Design review of the part shown in the three views and the two pictorial views. Dimensions are in mm from the part's minimum x, y and z. A direction names the side the tool comes from. Coordinates: 2 decimals unless noted, no trailing zeros. Loops run counter-clockwise (first coordinate to the right, second up) from the corner with the lowest first, then second, coordinate; pieces in that order, holes last. Notation, with made-up numbers: (-16, -14.75) -> (-4, -14.75) arc R11 ccw to (-4, -7.75) -> close; hole circle Ø9 at (71.25, 69). An arc over 180 degrees is marked (long way). One line per item, written item: value.
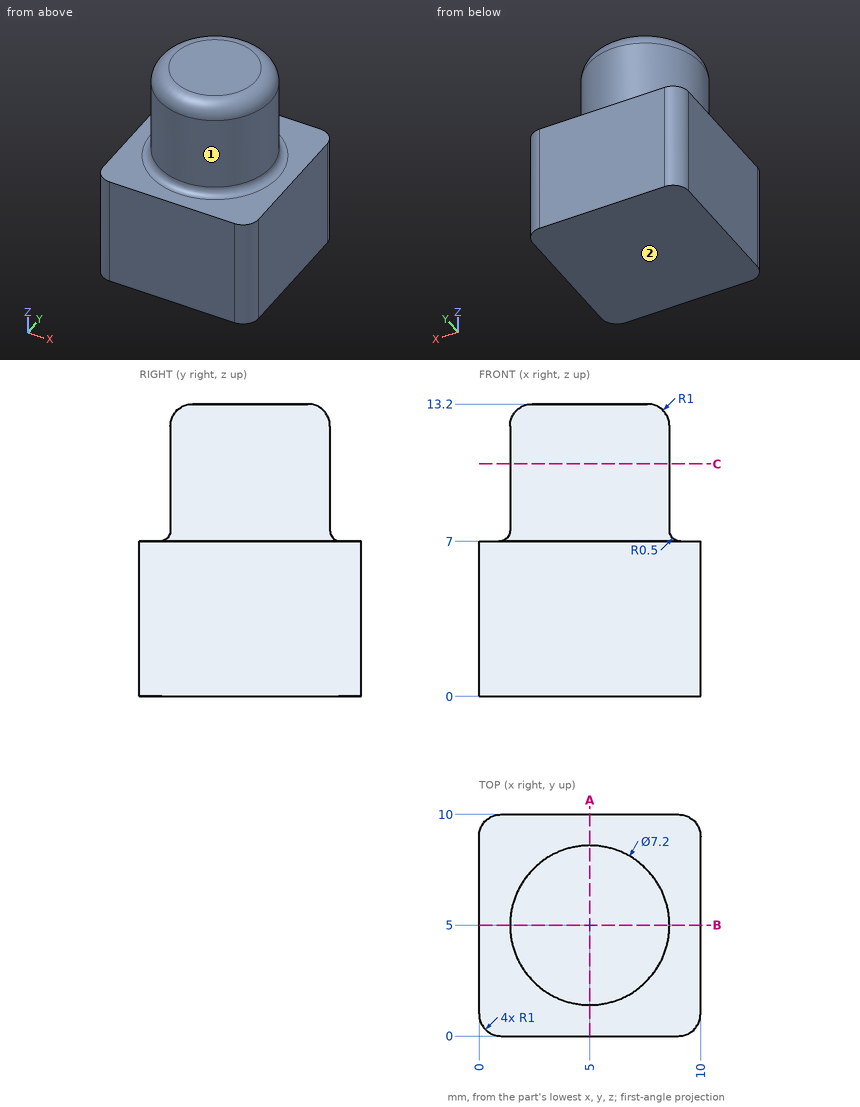
1. For the marked faces 1 and 2, list the 3-axis set-ups (+Z, -Z, +X, -X, +Y, -Y) from which the entire face can be reached by the end or side of a thin tool; tool diameter is ignored.
Return value:
face 1: +Z
face 2: -Z, +X, -X, +Y, -Y
2. Take a section at A-A, the plane x = 5. Give the boundary of the cut face in (y, z).
Return value:
outline: (0, 0) -> (10, 0) -> (10, 7) -> (9.1, 7) arc R0.5 cw to (8.6, 7.5) -> (8.6, 12.2) arc R1 ccw to (7.6, 13.2) -> (2.4, 13.2) arc R1 ccw to (1.4, 12.2) -> (1.4, 7.5) arc R0.5 cw to (0.9, 7) -> (0, 7) -> close
3. Insertion check: pin 1 Ø4 at (y, z) = (6.5, 10) entering from +X. The pin has a flat end and moves straight along its axis. Give the tip position at first contact, or say it passes through.
Return value:
pin 1: stops at x = 8.6
4. To check wall thickness, follow probe 1 along Z at (x, y) = (9.25, 8); probe 2 along X at (y, z) = (9.5, 4.75); probe 3 along X at (y, z) = (3.25, 7.75). State the ranges of each line that lie inside material, in increasing order. Write a range as from..to.
Return value:
probe 1: z = 0..7
probe 2: x = 0.13..9.87
probe 3: x = 1.85..8.15
5. Take a section at C-C, the plane z = 10.5. Give the boundary of the cut face in (x, y), and give its area (3 significant figures).
Return value:
outline: circle Ø7.2 at (5, 5)
area: 40.7 mm2
